Input: dimensioned drawing with shaded views. Units: mm. Origin: part minimum x, y, z. Round coordinates to 2 decimals unless told otherwise and drop trailing zeros.
1) Ray query, line 1 along X through (y, z) = (2, 10) (1 decimal); line 2 along Z through (x, y) = (54.5, 1) (1 decimal); line 3 along Z through (x, y) = (9, 5.5) (1 decimal). Return the intervals inside material, ascending.
2) First-contact query: pin 1 (6 mm diameter, centred on x = 11, z = 16, fed in from -Y) (1 decimal). Flat tip, straight axial feed; report the tip coordinate or a pass-through.
3) Draft query along Z for the marked faces 1, 2 and 3. Return one class per face: pulls with the +Z half, pulls with the -Z half, needs draft (parallel to the pull), parting line crosses it, or undercut.
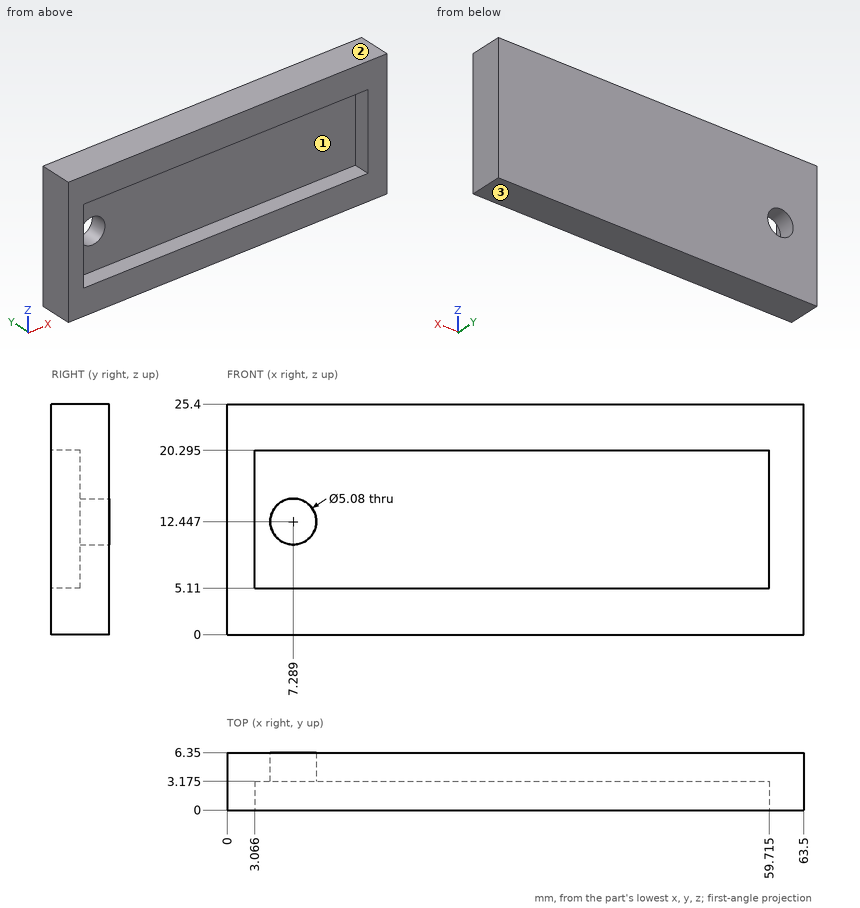
Final values:
1. line 1: x = 0 to 3.1, 59.7 to 63.5
1. line 2: z = 0 to 5.1, 20.3 to 25.4
1. line 3: z = 0 to 10.6, 14.3 to 25.4
2. pin 1: stops at y = 3.2
3. face 1: undercut
3. face 2: pulls with the +Z half
3. face 3: pulls with the -Z half
